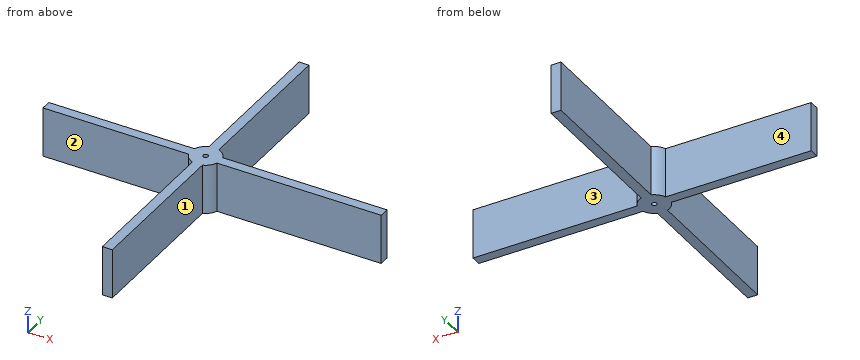
```python
from build123d import *

# Parameters (mm, degrees)
BOSS_EXTRUDE2_DEPTH      = 50
SKETCH2_R                = 15
BOSS_EXTRUDE3_DEPTH      = 50
F_5_0_5_DIAMETER_HOLE1_D = 5


with BuildPart() as part:
    # Sketch1 → Boss-Extrude2 (new body)
    with BuildSketch(Plane.XY):
        Polygon((-160.605737387, 5), (-5, 5), (-5, 170), (5, 170), (5, 5), (179.394262613, 5), (179.394262613, -5), (5, -5), (5, -170), (-5, -170), (-5, -5), (-160.605737387, -5), align=None)
    extrude(amount=BOSS_EXTRUDE2_DEPTH)

    # Sketch2 → Boss-Extrude3 (add)
    with BuildSketch(Plane(origin=(0, 0, 0), x_dir=(-1, 0, 0), z_dir=(0, 0, -1))):
        Circle(SKETCH2_R)
    extrude(amount=-BOSS_EXTRUDE3_DEPTH)

    # Ø5.0 (5) Diameter Hole1 (through all)
    with Locations(Plane.XY.offset(50)):
        with Locations((0, 0)):
            Hole(F_5_0_5_DIAMETER_HOLE1_D / 2)


solid = part.part
```
For this review, take the finished solid that the model builds, in its own axes (mm). Face numbers are marked on the shaded views. A direction names the side the tool comes from. Round coordinates to 2 decimals unless told otherwise and drop trailing zeros. Write each loop counter-clockwise with the first axis right and the second up, starting at its lowest first coordinate (ties: lowest second). Pieces come first, ordered by that corner, then holes. Notation, with made-up numbers: (-33.75, 68) - (10.25, 68) arc R20 ccw to (10.25, 102) - close; hole circle Ø2 at (12.25, 56.25). An arc over 180 degrees is marked (long way). Answer as a JSON object with one key per item and string values.
1. To check wall thickness, follow line 1 along Y through (x, z) = (0, 22.5); line 2 along X through (y, z) = (-104, 5). State the ranges of each line that lie inside material, in increasing order.
Response values:
{"line 1": "y = -170 to -2.5, 2.5 to 170", "line 2": "x = -5 to 5"}
2. We need section A-A on z = 16.5. Give the boundary of the cut face in (x, y).
Response values:
{"outline": "(-160.61, -5) - (-14.14, -5) arc R15 ccw to (-5, -14.14) - (-5, -170) - (5, -170) - (5, -14.14) arc R15 ccw to (14.14, -5) - (179.39, -5) - (179.39, 5) - (14.14, 5) arc R15 ccw to (5, 14.14) - (5, 170) - (-5, 170) - (-5, 14.14) arc R15 ccw to (-14.14, 5) - (-160.61, 5) - close; hole circle Ø5 at (0, 0)"}
3. For pin 1 Ø15 at (x, z) = (-120.5, 28) entering from +Y; pin 2 Ø5 at (y, z) = (-13, 17.5) entering from +X; pin 3 Ø15 at (y, z) = (-83, 14.5) entering from -X; pin 4 Ø6 at (x, y) = (0, 0) entering from +Z, all flat-tipped, find the tip position at first contact; note any pin that passes through.
Response values:
{"pin 1": "stops at y = 5", "pin 2": "stops at x = 10.71", "pin 3": "stops at x = -5", "pin 4": "stops at z = 50"}
4. Tool access review of the marked faces 1, 2, 3 and 4: name each direction out of +Z, -Z, +X, -X, +Y, -Y from which nothing blocks a thin tool from reaching the whole face with its end or side.
Response values:
{"face 1": "+Z, -Z, +X, -Y", "face 2": "+Z, -Z, -X, -Y", "face 3": "+Z, -Z, +X, +Y", "face 4": "+Z, -Z, -X, +Y"}
5. We need section B-B on x = 92.5. Give the boundary of the cut face in (y, z).
Response values:
{"outline": "(-5, 0) - (5, 0) - (5, 50) - (-5, 50) - close"}
